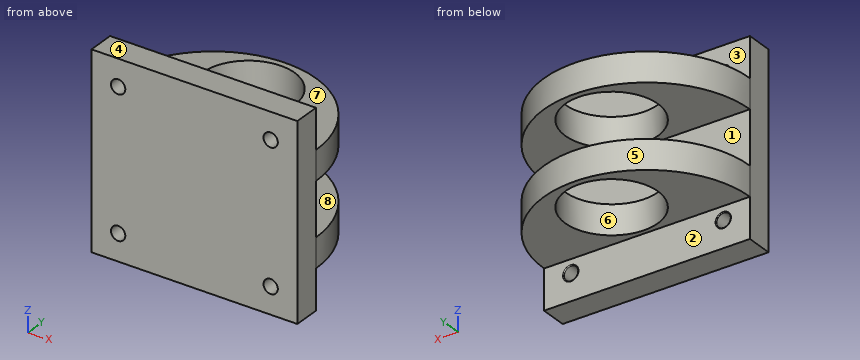
Autodesk Inventor part; units mm, degrees
ref_plane "Work Plane1" through (0, 0, -16.51) normal (0, 0, 1) x (1, 0, 0)
ref_plane "Work Plane2" through (0, 0, -22.86) normal (0, 0, 1) x (1, 0, 0)
ref_plane "YZ Plane" through (0, 0, 0) normal (1, 0, 0) x (0, 1, 0)
sketch "Sketch1" plane through (0, 0, 0) normal (0, 1, 0) x (-1, 0, 0)
  line L0 (0, 0) -> (-48.9966, 0)
  line L1 (-48.9966, 0) -> (-48.9966, -45.72)
  line L2 (-48.9966, -45.72) -> (0, -45.72)
  line L3 (0, -45.72) -> (0, 0)
  dimension "d0" = 48.9966
  dimension "d1" = 45.72
extrude "Extrusion1" add sketch "Sketch1" along normal blind 6.35
sketch "Sketch3" plane through (0, 6.35, 0) normal (0, 1, 0) x (1, 0, 0)
  line L0 (0, 45.72) -> (0, 0)
  line L1 (48.9966, 0) -> (48.9966, 45.72)
  line L2 (0, 29.21) -> (48.9966, 29.21)
  line L3 (48.9966, 29.21) -> (48.9966, 16.51)
  line L4 (48.9966, 16.51) -> (0, 16.51)
  line L5 (0, 16.51) -> (0, 29.21)
  line L6 (48.9966, 45.72) -> (0, 45.72)
  dimension "d4" = 12.7
  dimension "d5" = 16.51
sketch "Sketch4" plane through (0, 6.35, 0) normal (0, 1, 0) x (1, 0, 0)
  circle A0 centre (6.35, 39.37) radius 2.1364
  circle A1 centre (42.6466, 39.37) radius 3.0733
  line L0 (48.9966, 45.72) -> (0, 45.72)
  line L1 (48.9966, 0) -> (48.9966, 45.72)
  line L2 (0, 45.72) -> (0, 0)
  circle A2 centre (6.35, 6.35) radius 2.2799
  circle A3 centre (42.6466, 6.35) radius 1.194
  line L3 (0, 0) -> (48.9966, 0)
  dimension "d6" = 6.1465
  dimension "d7" = 6.35
  dimension "d8" = 6.35
  dimension "d9" = 6.35
  dimension "d10" = 6.35
  dimension "d11" = 6.35
  dimension "d12" = 6.35
  dimension "d13" = 6.35
  dimension "d14" = 6.35
hole "Hole1" at (6.35, 6.35, -39.37) at (42.6466, 6.35, -39.37) at (42.6466, 6.35, -6.35) at (6.35, 6.35, -6.35) direction (0, -1, 0) diameter 3.4 depth 10 tip angle 118
fillet "Fillet1" radius 0.2 4 edges at (42.6466, 6.35, -41.07) (6.35, 6.35, -41.07) (42.6466, 6.35, -8.05) (6.35, 6.35, -8.05)
ref_plane "Work Plane1" through (0, 0, -16.51) normal (0, 0, 1) x (1, 0, 0)
sketch "Sketch5" plane through (0, 0, -16.51) normal (0, 0, 1) x (1, 0, 0)
  line L0 (0, 6.35) -> (48.9966, 6.35)
  line L1 (48.9966, 6.35) -> (0, 6.35)
  arc A0 (48.9966, 6.35) -> (0, 6.35) centre (24.4983, 6.35) ccw
  point P0 (0, 0)
extrude "Extrusion2" add sketch "Sketch5" along normal blind 7
ref_plane "Work Plane2" through (0, 0, -22.86) normal (0, 0, 1) x (1, 0, 0)
mirror "Mirror1" about plane through (0, 0, -22.86) normal (0, 0, 1) of "Extrusion2"
sketch "Sketch6" plane through (0, 0, -9.51) normal (0, 0, 1) x (1, 0, 0)
  circle A0 centre (24.4983, 18.415) radius 11
  line L0 (0, 6.35) -> (48.9966, 6.35)
  point P0 (0, 0)
  point P1 (24.4983, 6.35)
  point P2 (24.4983, 6.35)
  dimension "d27" = 12.065
  dimension "d28" = 22
extrude "Extrusion3" cut sketch "Sketch6" against normal up to surface (7 mm away)
mirror "Mirror2" about plane through (0, 0, -22.86) normal (0, 0, 1) of "Extrusion3"
properties part number "Carriage Top Second Option" material "Aluminum 6061"
CAD build for the part. Positions are in the model's coordinates, mm. Face numbers are marked on the shaded views. A direction names the side the tool comes from. Coordinates: 2 decimals unless noted, no trailing zeros. Write each loop counter-clockwise with the first axis right and the second up, starting at its lowest first coordinate (ties: lowest second). Pieces come first, ordered by that corner, then holes. Notation, with made-up numbers: M 23.25,31 L 53.25,31 A27 ccw 53.25,57 Z; hole C -35,-32.5 d3. An arc over 180 degrees is marked long. Answer as a JSON object with one key per item and string values. Group by question number.
1) Saw through at B-B (y = 22.5). Write the cut outline in (x, z), plus the area to 3 significant figures.
2) Saw through at C-C (x = 6.35). Write the cut outline in (y, z).
3) Tool access for the marked faces 1, 2, 3, 4 and 5: list every direction of +Z, -Z, +X, -X, +Y, -Y with a clear straight run to the whole face (end or side of a thin tool).
4) Saw through at D-D (z = -32). Write the cut outline in (x, y) (3 decimals).
5) Wall check: line 1 (X direction, y = 3, z = -6.35); line 2 (Z direction, x = 6.35, y = 3.5); line 3 (Z direction, x = 47.5, y = 7). Give the ranges that are in metal, low to high. Write a range as from..to.
6) Mould opens along Z. For the marked faces 6, 7 and 8 say: +Z half, -Z half, draft (parallel to the pull), parting line (faces both ways), or undercut.
7) Saw through at A-A (z = -39.37). Write the cut outline in (x, y).
8) Pin check, flat tips, straight feed: pin 1 Ø6 at (y, z) = (25, -10.5) entering from +X; pin 2 Ø10.5 at (x, z) = (15.5, -5) entering from +Y; pin 3 Ø3 at (y, z) = (27.5, -36.5) entering from +X; pin 4 Ø2 at (x, z) = (6.35, -6.35) entering from +Y. Stop position of each tip, or through.
Values follow:
{
 "1": {"outline": "M 6.08,-36.21 L 14.28,-36.21 L 14.28,-29.21 L 6.08,-29.21 Z; M 6.08,-16.51 L 14.28,-16.51 L 14.28,-9.51 L 6.08,-9.51 Z; M 34.71,-36.21 L 42.92,-36.21 L 42.92,-29.21 L 34.71,-29.21 Z; M 34.71,-16.51 L 42.92,-16.51 L 42.92,-9.51 L 34.71,-9.51 Z", "area": "230 mm2"},
 "2": {"outline": "M 0,-45.72 L 6.35,-45.72 L 6.35,-41.27 A0.2 ccw 6.15,-41.07 L 0,-41.07 Z; M 0,-37.67 L 6.15,-37.67 A0.2 ccw 6.35,-37.47 L 6.35,-36.21 L 22.81,-36.21 L 22.81,-29.21 L 6.35,-29.21 L 6.35,-16.51 L 22.81,-16.51 L 22.81,-9.51 L 6.35,-9.51 L 6.35,-8.25 A0.2 ccw 6.15,-8.05 L 0,-8.05 Z; M 0,-4.65 L 6.15,-4.65 A0.2 ccw 6.35,-4.45 L 6.35,0 L 0,0 Z"},
 "3": {"face 1": "+X, -X, +Y", "face 2": "-Z, +X, -X, +Y", "face 3": "+Z, +X, -X, +Y", "face 4": "+Z, +X, -X, +Y, -Y", "face 5": "+Z, -Z, +Y"},
 "4": {"outline": "M 0,0 L 48.997,0 L 48.997,6.35 A24.498 ccw 0,6.35 Z; hole C 24.498,18.415 d22"},
 "5": {"line 1": "x = 0..4.65, 8.05..40.95, 44.35..49", "line 2": "z = -45.72..-41.07, -37.67..-8.05, -4.65..0", "line 3": "z = -36.21..-29.21, -16.51..-9.51"},
 "6": {"face 6": "draft", "face 7": "+Z half", "face 8": "undercut"},
 "7": {"outline": "M 0,0 L 4.65,0 L 4.65,6.15 A0.2 ccw 4.45,6.35 L 0,6.35 Z; M 8.05,0 L 40.95,0 L 40.95,6.15 A0.2 ccw 40.75,6.35 L 8.25,6.35 A0.2 ccw 8.05,6.15 Z; M 44.35,0 L 49,0 L 49,6.35 L 44.55,6.35 A0.2 ccw 44.35,6.15 Z"},
 "8": {"pin 1": "stops at x = 43.35", "pin 2": "stops at y = 30.02", "pin 3": "stops at x = 39.09", "pin 4": "passes through"}
}
